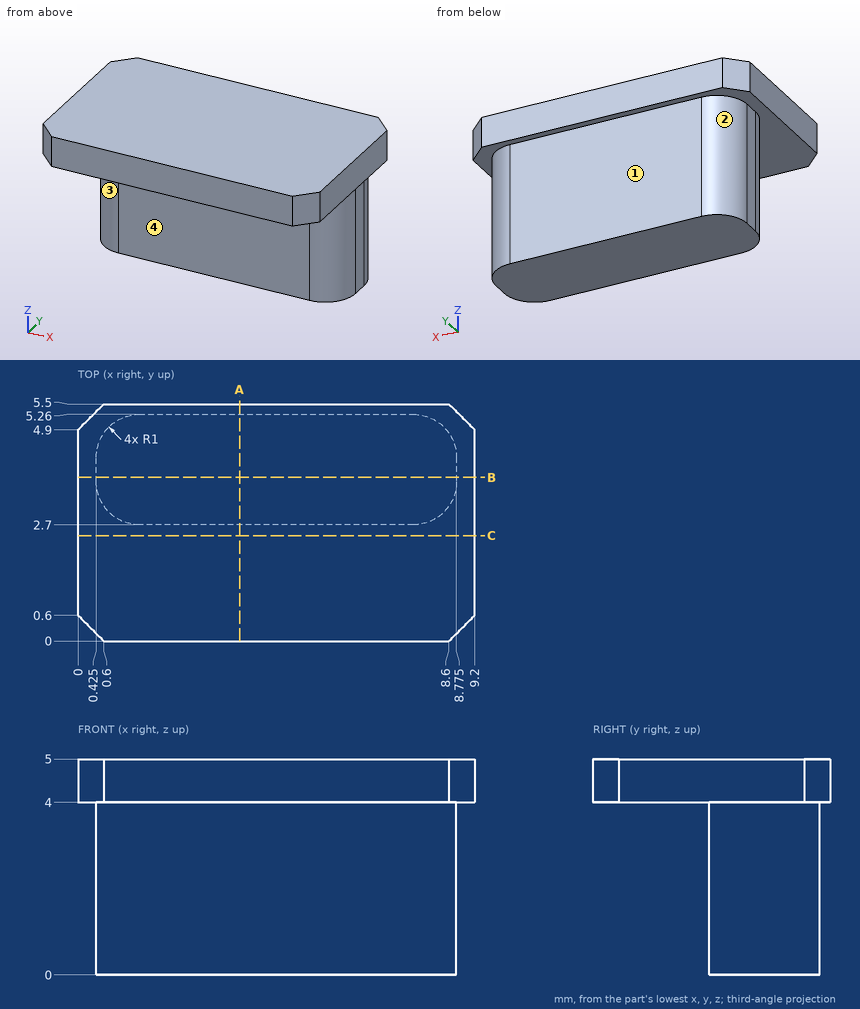
Drawing for the job (mm, zero at the part's lowest x, y, z). A direction names the side the tool comes from. Coordinates: 2 decimals unless noted, no trailing zeros. Write each loop counter-clockwise with the first axis right and the second up, starting at its lowest first coordinate (ties: lowest second). Pieces come first, ordered by that corner, then holes. Notation, with made-up numbers: (49.25, 63.5) - (56.25, 63.5) arc R20 ccw to (56.25, 67.5) - close; hole circle Ø3 at (55, 78.25). An arc over 180 degrees is marked (long way). Write each question's results on one line, items separated by ' | '. Start each with the question number.
1) Cut at A-A (x = 3.75). Write the cut outline in (y, z), then the cut area to 3 significant figures.
2) Flat gauge pins, fed straight in: P1, Ø0.6, axis at y = 4, z = 2.5, coming from the +X side (3 decimals); P2, Ø1.2, axis at x = 5, z = 1, coming from the -Y side; P3, Ø3, axis at x = 5.5, y = 0.5, coming from the -Z side; P4, Ø1.5, axis at y = 1, z = 1.5, coming from the -X side. Where does each tip first touch, or does it go through?
3) Cut at C-C (y = 2.45). Write the cut outline in (x, z), then the cut area to 3 significant figures.
4) 3-axis set-ups, long thin cutter, end or side, ignore diameter. For the marked faces 1, 2, 3 and 4: which of +Z, -Z, +X, -X, +Y, -Y reach the whole face in a straight line?
5) Cut at B-B (y = 3.8). Write the cut outline in (x, z) (3 decimals), then the cut area to 3 significant figures.
6) Probe line 1 along Z through (x, y) = (0.75, 1.8); line 2 along Y through (x, z) = (6, 1.35); line 3 along X through (y, z) = (4.25, 0.75) (3 decimals). List the from-to ranges inside material, lowest first. Write a range as from..to.
Returned:
1) outline: (0, 4) - (2.7, 4) - (2.7, 0) - (5.26, 0) - (5.26, 4) - (5.5, 4) - (5.5, 5) - (0, 5) - close | area: 15.7 mm^2
2) P1: x = 8.775 | P2: y = 2.7 | P3: z = 4 | P4: through
3) outline: (0, 4) - (9.2, 4) - (9.2, 5) - (0, 5) - close | area: 9.20 mm^2
4) face 1: -Z, +X, -X, +Y | face 2: -Z, -X, +Y | face 3: -Z, -X, -Y | face 4: -Z, +X, -X, -Y
5) outline: (0, 4) - (0.425, 4) - (0.425, 0) - (8.775, 0) - (8.775, 4) - (9.2, 4) - (9.2, 5) - (0, 5) - close | area: 42.6 mm^2
6) line 1: 4..5 | line 2: 2.7..5.26 | line 3: 0.425..8.775
